Study the drawing (mm; zero at the part's minimum x, y, z) and answer. Give positions to 0.01 mm unless a question says otherwise; leave off trailing zeros. Order: outer loops, then holes, each group sorted by start corner. A loop starts at its lowest first (then second) coordinate and runs counter-clockwise, first axis right, second up.
Item 1: A cutting plane is placed at C-C (z = 125.5). Write down the section's boundary in (x, y), plus the area to 3 significant figures.
Item 2: Given pin 1 Ø2 at (y, z) = (5, 132.5) entering from -X; pin 2 Ø3 at (y, z) = (3, 46) entering from -X, each flat-ended and moving along its own axis, determine where each tip first touches the part or whether it passes through.
Item 3: Find the intervals of material crossed by line 1 along X through (y, z) = (3.75, 18); line 2 along X through (y, z) = (5.3, 107) (1 decimal), in increasing order.
Item 4: A cutting plane is placed at B-B (x = 55). Write down the section's boundary in (y, z).
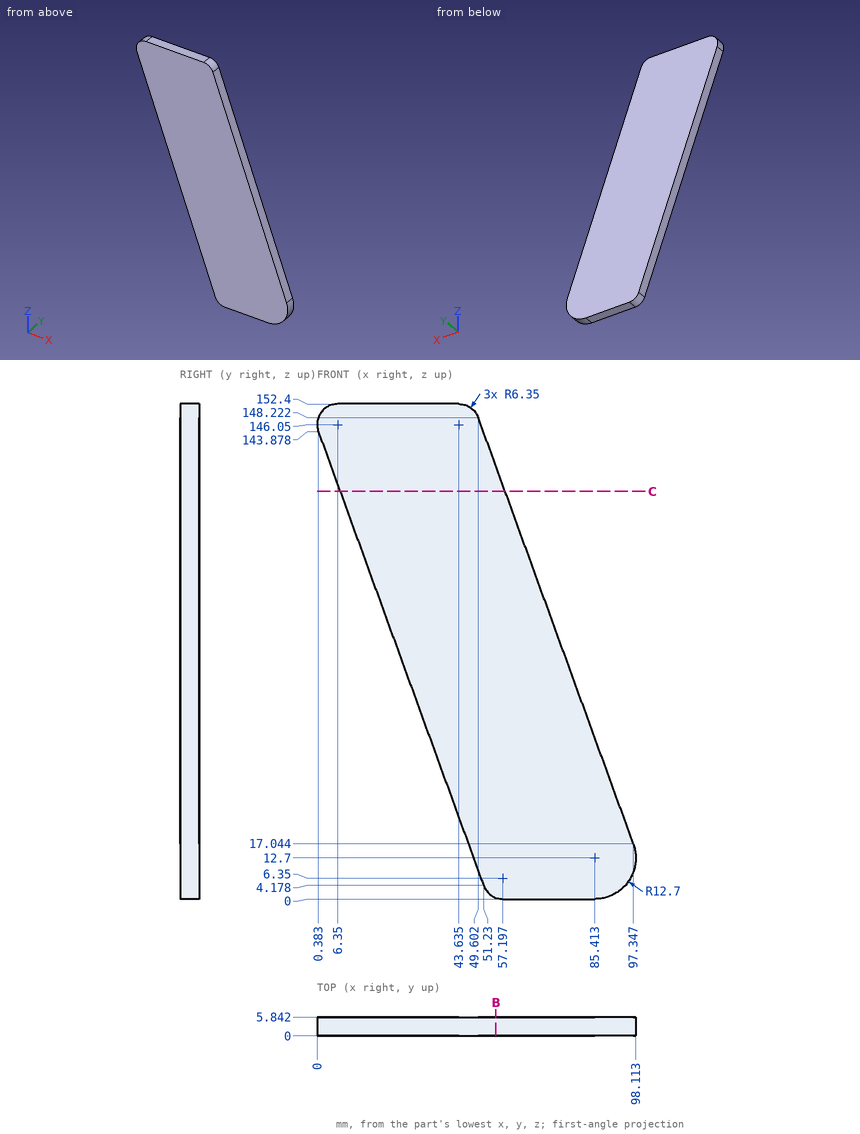
Response values:
1. outline: (7.07, 0) - (57.87, 0) - (57.87, 5.84) - (7.07, 5.84) - close
1. area: 297 mm2
2. pin 1: stops at x = 4.16
2. pin 2: stops at x = 35.46
3. line 1: x = 46.2 to 97
3. line 2: x = 13.8 to 64.6
4. outline: (0, 0.39) - (5.84, 0.39) - (5.84, 133.39) - (0, 133.39) - close
